Input: part model. Units: mm. Frame: model coordinates. A direction names the side the tool comes from. Give positions to 0.01 mm unless a question says otherwise; leave off trailing zeros. Write each loop counter-clockwise with the first axis right and the second up, starting at its lowest first coordinate (ties: lowest second). Pieces come first, ordered by that corner, then holes.
```python
from build123d import *

# Parameters (mm, degrees)
BOSS_EXTRUDE7_DEPTH = 5
SKETCH5_W           = 13.567085075
SKETCH5_H           = 3.932792286
BOSS_EXTRUDE8_DEPTH = 5
SKETCH6_W           = 50.2
SKETCH6_H           = 5
BOSS_EXTRUDE9_DEPTH = 25.2
SKETCH7_R           = 8.1
CUT_EXTRUDE1_DEPTH  = 10
CUT_EXTRUDE2_DEPTH  = 10
SKETCH9_R           = 1.6
CUT_EXTRUDE4_DEPTH  = 10


with BuildPart() as part:
    # Sketch1 → Boss-Extrude7 (new body)
    with BuildSketch(Plane(origin=(0, 0, 0), x_dir=(1, 0, 0), z_dir=(0, 1, 0))):
        Polygon((12.769214264, 6.275388257), (24.369214264, 6.275388257), (24.369214264, 0.275388257), (28.869214264, 0.275388257), (28.869214264, 6.275388257), (32.169214264, 6.275388257), (32.169214264, 0.275388257), (36.669214264, 0.275388257), (36.669214264, 6.275388257), (48.269214264, 6.275388257), (48.269214264, 21.275388257), (12.769214264, 21.275388257), align=None)
    extrude(amount=BOSS_EXTRUDE7_DEPTH)

    # Sketch5 → Boss-Extrude8 (add)
    with BuildSketch(Plane(origin=(0, 5, 0), x_dir=(1, 0, 0), z_dir=(0, 1, 0))):
        with Locations((30.552756802, 19.308992114)):
            Rectangle(SKETCH5_W, SKETCH5_H)
    extrude(amount=BOSS_EXTRUDE8_DEPTH)

    # Sketch6 → Boss-Extrude9 (add)
    with BuildSketch(Plane(origin=(1.124638213, 10, 0), x_dir=(1, 0, 0), z_dir=(0, 1, 0))):
        with Locations((29.394576051, 18.794771585)):
            Rectangle(SKETCH6_W, SKETCH6_H)
    extrude(amount=BOSS_EXTRUDE9_DEPTH)

    # Sketch7 → Cut-Extrude1 (cut)
    with BuildSketch(Plane.XY.offset(-16.294771585)):
        with Locations((17.119214264, 23.75)):
            Circle(SKETCH7_R)
        with Locations((43.619214264, 23.75)):
            Circle(SKETCH7_R)
    extrude(amount=-CUT_EXTRUDE1_DEPTH, mode=Mode.SUBTRACT)

    # Sketch7_3 → Cut-Extrude2 (cut)
    with BuildSketch(Plane.XY.offset(-16.294771585)):
        with BuildLine():
            Line((26.566421185, 18.4), (33.366421185, 18.4))
            ThreePointArc((33.366421185, 18.4), (35.566421185, 16.2), (33.366421185, 14))
            Line((33.366421185, 14), (26.566421185, 14))
            ThreePointArc((26.566421185, 14), (24.366421185, 16.2), (26.566421185, 18.4))
        make_face()
    extrude(amount=-CUT_EXTRUDE2_DEPTH, mode=Mode.SUBTRACT)

    # Sketch9 → Cut-Extrude4 (cut)
    with BuildSketch(Plane(origin=(0, 5, 0), x_dir=(1, 0, 0), z_dir=(0, 1, 0))):
        with Locations((26.619214264, 3.275388257)):
            Circle(SKETCH9_R)
        with Locations((34.419214264, 3.275388257)):
            Circle(SKETCH9_R)
    extrude(amount=-CUT_EXTRUDE4_DEPTH, mode=Mode.SUBTRACT)


solid = part.part
```
Item 1: Section A-A (y = 23.75). Return loops of the section in (x, z), and give its area (3 significant figures).
Item 2: Set-up query: faces 1 (the flat face through (18, 2, -6.275)), 2 (the flat face through (42, 2, -6.275)), 3 (the flat face through (28.869, 2, -3)). Return all of +Z, -Z, +X, -X, +Y, -Y with unobstructed straight access to the full face (end or side cutting, diameter ignored); none if empty.
Item 3: Pin query (flat end, axial travel): pin 1 (2.5 mm diameter, centred on y = 2.5, z = -2, fed in from +X); pin 2 (3 mm diameter, centred on x = 28, y = 3, fed in from -Z); pin 3 (2.5 mm diameter, centred on x = 19, y = 1.5, fed in from +Z); pin 4 (1.5 mm diameter, centred on y = 6.5, z = -13.5, fed in from +X) (3 decimals). Return the tip coordinate at first contact, or that it passes through.
Item 4: Ray query, line 1 (Y direction, x = 32.5, z = -17); line 2 (Y direction, x = 13, z = -20.25); line 3 (X direction, y = 21.5, z = -19.75). Return the intervals inside material, ascending.
Item 5: Mould query, pull axis Y, two halves, no side actions, for faces 4 (the flat face through (30, 7, -17.343)), 5 (the flat face through (30, 0, -13)), 6 (the flat face through (30, 14, -19)), 7 (the flat face through (48.269, 2, -14)). Classes: +Y half, -Y half, draft (parallel to the pull), parting line (faces both ways), or undercut.
Item 6: Section D-D (y = 16.2). Return loops of the section in (x, z).
Item 7: Section C-C (x = 14.5). Return loops of the section in (y, z).
Item 8: Section B-B (z = -5.75). Return loops of the section in (x, y).
Solved:
1. outline: (5.42, -21.29) - (9.02, -21.29) - (9.02, -16.29) - (5.42, -16.29) - close; (25.22, -21.29) - (35.52, -21.29) - (35.52, -16.29) - (25.22, -16.29) - close; (51.72, -21.29) - (55.62, -21.29) - (55.62, -16.29) - (51.72, -16.29) - close
1. area: 89.0 mm2
2. face 1: +Z, -X, +Y, -Y
2. face 2: +Z, +X, +Y, -Y
2. face 3: +Z, +Y, -Y
3. pin 1: stops at x = 36.67
3. pin 2: stops at z = -21.28
3. pin 3: stops at z = -6.28
3. pin 4: passes through
4. line 1: y = 0 to 5, 10 to 14, 18.4 to 35.2
4. line 2: y = 0 to 5, 10 to 16.78, 30.72 to 35.2
4. line 3: x = 5.42 to 9.34, 24.9 to 35.84, 51.4 to 55.62
5. face 4: undercut
5. face 5: -Y half
5. face 6: undercut
5. face 7: draft
6. outline: (5.42, -21.29) - (14.19, -21.29) - (14.19, -16.29) - (5.42, -16.29) - close; (20.05, -21.29) - (24.37, -21.29) - (24.37, -16.29) - (20.05, -16.29) - close; (35.57, -21.29) - (40.69, -21.29) - (40.69, -16.29) - (35.57, -16.29) - close; (46.55, -21.29) - (55.62, -21.29) - (55.62, -16.29) - (46.55, -16.29) - close
7. outline: (0, -21.28) - (5, -21.28) - (5, -6.28) - (0, -6.28) - close; (10, -21.29) - (16.09, -21.29) - (16.09, -16.29) - (10, -16.29) - close; (31.41, -21.29) - (35.2, -21.29) - (35.2, -16.29) - (31.41, -16.29) - close
8. outline: (24.37, 0) - (28.87, 0) - (28.87, 5) - (24.37, 5) - close; (32.17, 0) - (36.67, 0) - (36.67, 5) - (32.17, 5) - close
